```python
from build123d import *

# Parameters (mm, degrees)
F1_DEPTH = 19.05
F2_W     = 44.45
F2_H     = 19.05
F3_DEPTH = 63.5
F5_DEPTH = 19.05


with BuildPart() as f1:
    # F0 (on Right) → F1 (new body)
    with BuildSketch(Plane.YZ):
        Polygon((14.978143, 21.367056), (-4.071857, 21.367056), (-48.521857, -10.382944), (-48.521857, -23.082944), (14.978143, -23.082944), align=None)
    extrude(amount=F1_DEPTH)

    # F2 (on face) → F3 (join)
    with BuildSketch(Plane(origin=(0, 0, 0), x_dir=(0, -1, 0), z_dir=(-1, 0, 0))):
        with Locations((7.246857, -13.557944)):
            Rectangle(F2_W, F2_H)
    extrude(amount=F3_DEPTH)

    # F4 (on face) → F5 (join)
    with BuildSketch(Plane(origin=(-63.5, 0, 0), x_dir=(0, -1, 0), z_dir=(-1, 0, 0))):
        Polygon((-13.703029, 21.348763), (-14.978143, -23.082944), (48.521857, -23.082944), (48.521857, -10.382944), (5.346971, 21.348763), align=None)
    extrude(amount=F5_DEPTH)


solid = f1.part
```
The listing builds one solid part. Answer for the finished solid, in the listing's coordinates (mm). A direction names the side the tool comes from. Coordinates: 2 decimals unless noted, no trailing zeros. Loops run counter-clockwise (first coordinate to the right, second up) from the corner with the lowest first, then second, coordinate; pieces in that order, holes last. Notation, with made-up numbers: M 17,77.5 L 39,77.5 A30 ccw 39,99.5 Z; hole C 75,51 d3. An arc over 180 degrees is marked long. Answer as a JSON object with one key per item and string values. Group by question number.
Item 1: Section C-C (x = -69.5) is taken. Write down the section's boundary in (y, z).
Item 2: Section B-B (y = -43.5) is taken. Write down the section's boundary in (x, z).
Item 3: Section D-D (y = -18.5) is taken. Write down the section's boundary in (x, z).
Item 4: Determine the mould class of faces 1 (the face through (-73, -48.522, -17)), 2 (the face through (-63.5, -17, -1)), 3 (the face through (-82.55, -9, -5)), 4 (the face through (-31, -29.472, -14)) for opening direction X: +X half, -X half, draft (parallel to the pull), parting line (faces both ways), or undercut.
Item 5: Each of these flat-tipped pins is pushed along its axis until it touches: P1, Ø12, axis at x = -62.5, y = -20.5, coming from the +Z side; P2, Ø13.5, axis at x = -31.5, y = -18, coming from the +Z side; P3, Ø5.5, axis at x = -39.5, z = -14, coming from the -Y side. Where does it stop, or does it pass through?
Item 6: Section A-A (z = 8) is taken. Write down the section's boundary in (x, y).
Item 7: Which of the six approach directions +Z, -Z, +X, -X, +Y, -Y give full straight-line access (tool end or side, diameter ignored) to faces 5 (the face through (0, -17, -1)), 6 (the face through (9, 6, 21.367)), 7 (the face through (9.39, -25.99, 5.71)), 8 (the face through (-31, -7, -4.033)), 9 (the face through (9, -48.522, -17))?
Item 8: Consider L1, parallel to X at y = -2.5, z = 9.5; L2, parallel to Z at x = -36, y = -16; L3, parallel to Y at x = -52, z = -9.5. Determine where each line is inside the solid, lowest interval first.
Solved:
{
 "1": {"outline": "M -48.52,-23.08 L 14.98,-23.08 L 13.7,21.35 L -5.35,21.35 L -48.52,-10.38 Z"},
 "2": {"outline": "M -82.55,-23.08 L -63.5,-23.08 L -63.5,-6.69 L -82.55,-6.69 Z; M 0,-23.08 L 19.05,-23.08 L 19.05,-6.8 L 0,-6.8 Z"},
 "3": {"outline": "M -82.55,-23.08 L 19.05,-23.08 L 19.05,11.06 L 0,11.06 L 0,-4.03 L -63.5,-4.03 L -63.5,11.68 L -82.55,11.68 Z"},
 "4": {"face 1": "draft", "face 2": "undercut", "face 3": "-X half", "face 4": "undercut"},
 "5": {"P1": "stops at z = 14.56", "P2": "stops at z = -4.03", "P3": "stops at y = -29.47"},
 "6": {"outline": "M -82.55,-23.51 L -63.5,-23.51 L -63.5,14.09 L -82.55,14.09 Z; M 0,-22.79 L 19.05,-22.79 L 19.05,14.98 L 0,14.98 Z"},
 "7": {"face 5": "+Z, -Y", "face 6": "+Z, +X, -X, +Y, -Y", "face 7": "+Z, +X, -Y", "face 8": "+Z, +Y, -Y", "face 9": "+Z, -Z, +X, -X, -Y"},
 "8": {"L1": "x = -82.55 to -63.5, 0 to 19.05", "L2": "z = -23.08 to -4.03", "L3": "y = -29.47 to 14.98"}
}
